The listing builds one solid part. Answer for the finished solid, in the listing's coordinates (mm). A direction names the side the tool comes from. Coordinates: 2 decimals unless noted, no trailing zeros. Order: outer loops, then holes, each group sorted by start corner. A loop starts at its lowest first (then second) coordinate and runs counter-clockwise, first axis right, second up. Notation, with made-up numbers: (31, -16) -> (65, -16) arc R17 ccw to (65, 8) -> close; hole circle Ø1 at (10, 44). An arc over 180 degrees is marked (long way). Write item = value, one per line.
from build123d import *

# Parameters (mm, degrees)
EXTRUDE_THIN1_OUTLINE_W = 9
EXTRUDE_THIN1_OUTLINE_H = 12.5
EXTRUDE_THIN1_DEPTH     = 3.5
SKETCH1_3_W             = 10
SKETCH1_3_H             = 13.5
BOSS_EXTRUDE1_DEPTH     = 3.5
BOSS_EXTRUDE2_DEPTH     = 7
CUT_EXTRUDE1_DEPTH      = 39.801707437
CUT_EXTRUDE1_DEPTH_BACK = 39.801707437


# Read off the part's stored shape, not the designer's step: Extrude-Thin1
with BuildPart() as part:
    # Extrude-Thin1 outline → Extrude-Thin1 (new body)
    with BuildSketch(Plane.XY):
        with BuildLine():
            ThreePointArc((0.177562937, 22), (1.247898439, 19.536389911), (3.521526088, 18.106141657))
            Line((3.521526088, 18.106141657), (8.11763809, 16.874617158))
            ThreePointArc((8.11763809, 16.874617158), (9.6, 14.942765505), (8.11763809, 13.010913852))
            Line((8.11763809, 13.010913852), (2.923542865, 11.619160231))
            ThreePointArc((2.923542865, 11.619160231), (0.7, 8.721382753), (2.923542865, 5.823605274))
            Line((2.923542865, 5.823605274), (8.11763809, 4.431851653))
            ThreePointArc((8.11763809, 4.431851653), (9.582889723, 2.238947616), (7.6, 0.5))
            Line((7.6, 0.5), (0.65, 0.5))
            Line((0.65, 0.5), (0.65, -0.5))
            Line((0.65, -0.5), (7.6, -0.5))
            ThreePointArc((7.6, -0.5), (10.574334584, 2.108421424), (8.376457135, 5.397777479))
            Line((8.376457135, 5.397777479), (3.18236191, 6.7895311))
            ThreePointArc((3.18236191, 6.7895311), (1.7, 8.721382752), (3.18236191, 10.653234405))
            Line((3.18236191, 10.653234405), (8.376457135, 12.044988026))
            ThreePointArc((8.376457135, 12.044988026), (10.6, 14.942765505), (8.376457135, 17.840542984))
            Line((8.376457135, 17.840542984), (3.780345133, 19.072067483))
            ThreePointArc((3.780345133, 19.072067483), (2.042960507, 20.146152168), (1.185399159, 22))
            Line((1.185399159, 22), (11.15, 22))
            Line((11.15, 22), (11.15, 36.5))
            Line((11.15, 36.5), (0.15, 36.5))
            Line((0.15, 36.5), (0.15, 22))
            Line((0.15, 22), (0.177562937, 22))
        make_face()
        with Locations((5.65, 29.25)):
            Rectangle(EXTRUDE_THIN1_OUTLINE_W, EXTRUDE_THIN1_OUTLINE_H, mode=Mode.SUBTRACT)
    extrude(amount=EXTRUDE_THIN1_DEPTH)

    # Sketch1<3> → Boss-Extrude1 (add)
    with BuildSketch(Plane.XY):
        with Locations((5.65, 29.25)):
            Rectangle(SKETCH1_3_W, SKETCH1_3_H)
    extrude(amount=BOSS_EXTRUDE1_DEPTH)

    # Sketch2 → Boss-Extrude2 (add)
    with BuildSketch(Plane.XY.offset(3.5)):
        with BuildLine():
            Line((7.15, 26.5), (7.15, 23.5))
            ThreePointArc((7.15, 23.5), (5.65, 22), (4.15, 23.5))
            Line((4.15, 23.5), (4.15, 26.5))
            ThreePointArc((4.15, 26.5), (5.65, 28), (7.15, 26.5))
        make_face()
    extrude(amount=BOSS_EXTRUDE2_DEPTH)

    # Sketch3 → Cut-Extrude1 (cut, two sides: drawn at the far end of the back side and taken through both)
    with BuildSketch(Plane.XY.offset(3.5).offset(-CUT_EXTRUDE1_DEPTH_BACK)):
        Polygon((0.15, 26.5), (1.15, 28.5), (1.15, 36.7), (10.15, 36.7), (10.15, 28.636121044), (11.15, 26.5), (15.293937853, 34.999866887), (13.289839187, 39.280864223), (-0.624731021, 39.280864223), (-5.238216118, 36.366540163), align=None)
    extrude(amount=CUT_EXTRUDE1_DEPTH + CUT_EXTRUDE1_DEPTH_BACK, mode=Mode.SUBTRACT)


solid = part.part
Q1. Section A-A, the plane x = 5 is taken. Give the vertices of the cut face in (y, z).
The answers:
outline = (-0.5, 0) -> (0.5, 0) -> (0.5, 3.5) -> (-0.5, 3.5) -> close; (5.27, 0) -> (6.3, 0) -> (6.3, 3.5) -> (5.27, 3.5) -> close; (11.14, 0) -> (12.18, 0) -> (12.18, 3.5) -> (11.14, 3.5) -> close; (17.71, 0) -> (18.75, 0) -> (18.75, 3.5) -> (17.71, 3.5) -> close; (22, 0) -> (36.5, 0) -> (36.5, 3.5) -> (27.85, 3.5) -> (27.85, 10.5) -> (22.15, 10.5) -> (22.15, 3.5) -> (22, 3.5) -> close
Q2. A tool of negligible diameter and unlimited length cuts with its end or side. For faces 1 (the face through (1.15, 32, 2)), 2 (the face through (5.557, 12.325, 1.726)), 3 (the face through (4.15, 25, 7)), 4 (the face through (5.74, 11.34, 1.73)), 5 (the face through (7.15, 25, 7)), from which of +Z, -Z, +X, -X, +Y, -Y can it reach the whole face along a straight path? Write none if from no direction.
The answers:
face_1 = +Z, -Z, -X, +Y
face_2 = +Z, -Z, -X
face_3 = +Z, -X, +Y, -Y
face_4 = +Z, -Z, +X
face_5 = +Z, +X, +Y, -Y
Q3. The mould has two halves that part along Y. Classify faces 6 (the face through (0.15, 24, 2)), 7 (the face through (0.7, 8.8, 1.7)), 8 (the face through (6, 36.5, 2)), 9 (the face through (5.7, 22, 7)): released by +Y, released by -Y, zero draft, split by the parting line, or undercut.
The answers:
face_6 = zero draft
face_7 = undercut
face_8 = released by +Y
face_9 = released by -Y
Q4. Section D-D, the plane y = 32 is taken. Give the vertices of the cut face in (x, z), plus the area to 3 significant figures.
The answers:
outline = (1.15, 0) -> (10.15, 0) -> (10.15, 3.5) -> (1.15, 3.5) -> close
area = 31.5 mm2
Q5. Section B-B, the plane z = 6 is taken. Give the vertices of the cut face in (x, y), plus the area to 3 significant figures.
The answers:
outline = (4.15, 23.5) arc R1.5 ccw to (7.15, 23.5) -> (7.15, 26.5) arc R1.5 ccw to (4.15, 26.5) -> close
area = 16.1 mm2
Q6. Section C-C, the plane x = 2.25 is taken. Give the vertices of the cut face in (y, z).
The answers:
outline = (-0.5, 0) -> (0.5, 0) -> (0.5, 3.5) -> (-0.5, 3.5) -> close; (6.1, 0) -> (7.34, 0) -> (7.34, 3.5) -> (6.1, 3.5) -> close; (10.1, 0) -> (11.35, 0) -> (11.35, 3.5) -> (10.1, 3.5) -> close; (18.67, 0) -> (19.93, 0) -> (19.93, 3.5) -> (18.67, 3.5) -> close; (22, 0) -> (36.5, 0) -> (36.5, 3.5) -> (22, 3.5) -> close
Q7. Find the intervals of material crossed by line 1 along Y through (x, z) = (6, 2); line 2 along Y through (x, z) = (5, 2.75); line 3 along Z through (x, y) = (9.75, 17), in increasing order.
The answers:
line_1 = -0.5 to 0.5, 5 to 6.03, 11.41 to 12.44, 17.44 to 18.48, 22 to 36.5
line_2 = -0.5 to 0.5, 5.27 to 6.3, 11.14 to 12.18, 17.71 to 18.75, 22 to 36.5
line_3 = 0 to 3.5
Q8. Each of these flat-tipped pins is pushed along its axis until it touches: pin 1 Ø6 at (x, z) = (8.5, 4) entering from -Y; pin 2 Ø3.5 at (y, z) = (25, 8.5) entering from -X; pin 3 Ø3 at (y, z) = (34, 1) entering from -X; pin 4 Ø2.5 at (y, z) = (25, 6) entering from +X. Where does it stop, or does it pass through?
The answers:
pin_1 = -0.5
pin_2 = 4.15
pin_3 = 1.15
pin_4 = 7.15
